```python
from build123d import *

# Parameters (mm, degrees)
SKETCH1_W           = 30
SKETCH1_H           = 30
BOSS_EXTRUDE1_DEPTH = 12
SKETCH2_R           = 1.5
CUT_EXTRUDE1_DEPTH  = 45.09081537
SKETCH3_R           = 1.5
CUT_EXTRUDE2_DEPTH  = 5


with BuildPart() as part:
    # Sketch1 → Boss-Extrude1 (new body)
    with BuildSketch(Plane.XY):
        with Locations((15, 15)):
            Rectangle(SKETCH1_W, SKETCH1_H)
    extrude(amount=BOSS_EXTRUDE1_DEPTH)

    # Sketch2 → Cut-Extrude1 (cut, through all)
    with BuildSketch(Plane.XY.offset(12)):
        with Locations((5, 6)):
            Circle(SKETCH2_R)
        with Locations(Location((25, 6, 0), (0, 0, 180))):
            Circle(SKETCH2_R)
    extrude(amount=-CUT_EXTRUDE1_DEPTH, mode=Mode.SUBTRACT)

    # Sketch3 → Cut-Extrude2 (cut)
    with BuildSketch(Plane(origin=(0, 30, 0), x_dir=(1, 0, 0), z_dir=(0, 1, 0))):
        with Locations(Location((5, -6, 0), (0, 0, 270))):
            Circle(SKETCH3_R)
        with Locations(Location((25, -6, 0), (0, 0, 90))):
            Circle(SKETCH3_R)
    extrude(amount=-CUT_EXTRUDE2_DEPTH, mode=Mode.SUBTRACT)


solid = part.part
```
Source: CAD feature listing. Evaluate the final solid. Frame: model axes, mm. A direction names the side the tool comes from. Round coordinates to 2 decimals unless told otherwise and drop trailing zeros. Loops run counter-clockwise (first coordinate to the right, second up) from the corner with the lowest first, then second, coordinate; pieces in that order, holes last. Notation, with made-up numbers: M 29.5,-37 L 84.5,-37 A20 cw 84.5,-9 Z; hole C 16,44.5 d8. An arc over 180 degrees is marked long. Use a Markdown table: item, result. Add a question column.
1. Pull-direction query (Z, two-part tool) for faces 3 (the flat face through (15, 15, 12)), 4 (the flat face through (25, 25, 6)), 5 (the flat face through (15, 0, 6)); classes: +Z half, -Z half, draft (parallel to the pull), parting line (faces both ways), or undercut.
2. Cut plane A-A, the plane x = 25. Output: boundary loops of the cut face in (y, z), and give its area (3 significant figures).
3. Cut plane C-C, the plane z = 1. Output: boundary loops of the cut face in (x, y).
4. Cut plane B-B, the plane y = 6. Output: boundary loops of the cut face in (x, z), and give its area (3 significant figures).
5. Set-up query: faces 1 (the cylindrical face through (6.386, 5.425, 6.084)), 2 (the cylindrical face through (23.513, 27.535, 6.195)). Return all of +Z, -Z, +X, -X, +Y, -Y with unobstructed straight access to the full face (end or side cutting, diameter ignored); none if empty.
6. Contact query for flat-ended pins moving along their axis: pin 1 (1.8 mm diameter, centred on x = 25, y = 6, fed in from -Z); pin 2 (0.9 mm diameter, centred on x = 5, z = 6.5, fed in from +Y). Output: stop coordinate, or through.
7. Ray query, line 1 along X through (y, z) = (28.05, 6); line 2 along Y through (x, z) = (25, 4.75); line 3 along Y through (x, z) = (23.75, 7.25). Return the intervals inside material, ascending. Write a range as [from, to].
8. Cut plane D-D, the plane y = 27. Output: boundary loops of the cut face in (x, z).
Solution:
| question | item | result |
|---|---|---|
| 1 | face 3 | +Z half |
| 1 | face 4 | undercut |
| 1 | face 5 | draft |
| 2 | outline | M 0,0 L 4.5,0 L 4.5,12 L 0,12 Z; M 7.5,0 L 30,0 L 30,4.5 L 25,4.5 L 25,7.5 L 30,7.5 L 30,12 L 7.5,12 Z |
| 2 | area | 309 mm2 |
| 3 | outline | M 0,0 L 30,0 L 30,30 L 0,30 Z; hole C 5,6 d3; hole C 25,6 d3 |
| 4 | outline | M 0,0 L 3.5,0 L 3.5,12 L 0,12 Z; M 6.5,0 L 23.5,0 L 23.5,12 L 6.5,12 Z; M 26.5,0 L 30,0 L 30,12 L 26.5,12 Z |
| 4 | area | 288 mm2 |
| 5 | face 1 | +Z, -Z |
| 5 | face 2 | +Y |
| 6 | pin 1 | passes through |
| 6 | pin 2 | stops at y = 25 |
| 7 | line 1 | x = [0, 3.5], [6.5, 23.5], [26.5, 30] |
| 7 | line 2 | y = [0, 4.5], [7.5, 25] |
| 7 | line 3 | y = [0, 5.17], [6.83, 30] |
| 8 | outline | M 0,0 L 30,0 L 30,12 L 0,12 Z; hole C 5,6 d3; hole C 25,6 d3 |
